```python
from build123d import *

# Parameters (mm, degrees)
SKETCH1_W           = 64.2
SKETCH1_H           = 8.2
SKETCH1_W_2         = 61
SKETCH1_H_2         = 5
BOSS_EXTRUDE1_DEPTH = 90
SKETCH2_W           = 4
SKETCH2_H           = 8.2
BOSS_EXTRUDE2_DEPTH = 2
BOSS_EXTRUDE4_DEPTH = 8
SKETCH5_W           = 17.2
SKETCH5_H           = 27.6
BOSS_EXTRUDE5_DEPTH = 1.6
CHAMFER3_SIZE       = 11
FILLET1_R           = 3
FILLET2_R           = 2
FILLET3_R           = 3
SKETCH3_W           = 10
SKETCH3_H           = 10
BOSS_EXTRUDE3_DEPTH = 0.8


with BuildPart() as part:
    # Sketch1 → Boss-Extrude1 (new body)
    with BuildSketch(Plane.XY):
        Rectangle(SKETCH1_W, SKETCH1_H)
        Rectangle(SKETCH1_W_2, SKETCH1_H_2, mode=Mode.SUBTRACT)
    extrude(amount=BOSS_EXTRUDE1_DEPTH)

    # Sketch2 → Boss-Extrude2 (add)
    with BuildSketch(Plane(origin=(0, 0, 0), x_dir=(-1, 0, 0), z_dir=(0, 0, -1))):
        Rectangle(SKETCH2_W, SKETCH2_H)
    extrude(amount=-BOSS_EXTRUDE2_DEPTH)

    # Sketch4 → Boss-Extrude4 (add)
    with BuildSketch(Plane.XZ.offset(4.1)):
        Polygon((-7, 52.6), (-7, 26.6), (7, 26.6), (7, 52.6), (8.6, 52.6), (8.6, 25), (-8.6, 25), (-8.6, 52.6), align=None)
    extrude(amount=BOSS_EXTRUDE4_DEPTH)

    # Sketch5 → Boss-Extrude5 (add)
    with BuildSketch(Plane.XZ.offset(12.1)):
        with Locations((0, 38.8)):
            Rectangle(SKETCH5_W, SKETCH5_H)
    extrude(amount=BOSS_EXTRUDE5_DEPTH)

    # Chamfer3
    # the kernel refuses this chamfer: 11 mm, written as the material it adds along each edge
    with BuildSketch(Plane(origin=(8.6, -4.1, 25), x_dir=(0, 0.027495876610586372, -0.9996219169112968), z_dir=(-1, 0, 0))) as chamfer3_piece_1_section:
        Polygon((CHAMFER3_SIZE * 0.999621916911, CHAMFER3_SIZE * 0.0274958766106), (-CHAMFER3_SIZE * 0.0274958766106, CHAMFER3_SIZE * 0.999621916911), (0, 0), align=None)
    chamfer3_piece_1 = extrude(amount=17.2, mode=Mode.PRIVATE)
    chamfer3_piece_1 = split(chamfer3_piece_1, bisect_by=Plane(origin=(0, -13.7, 21.279882352), z_dir=(0, 1, 0)), keep=Keep.TOP, mode=Mode.PRIVATE)
    add(chamfer3_piece_1)

    # Fillet1
    fillet1_edges = [part.edges().sort_by_distance(p)[0] for p in [
        (-8.6, -4.1, 33.3),
        (8.6, -4.1, 33.3),
    ]]
    fillet(fillet1_edges, radius=FILLET1_R)

    # Fillet2
    fillet2_edges = [part.edges().sort_by_distance(p)[0] for p in [
        (2, -2.5, 1),
        (-2, -2.5, 1),
        (-2, 2.5, 1),
        (2, 2.5, 1),
    ]]
    fillet(fillet2_edges, radius=FILLET2_R)

    # Fillet3
    fillet3_edges = [part.edges().sort_by_distance(p)[0] for p in [
        (-9.3, -4.1, 52.6),
        (9.3, -4.1, 52.6),
    ]]
    fillet(fillet3_edges, radius=FILLET3_R)

    # Sketch3 → Boss-Extrude3 (add)
    with BuildSketch(Plane(origin=(0, 0, 0), x_dir=(-1, 0, 0), z_dir=(0, 0, -1))):
        with Locations((-35.5, 9.1)):
            Rectangle(SKETCH3_W, SKETCH3_H)
        with Locations((35.5, 9.1)):
            Rectangle(SKETCH3_W, SKETCH3_H)
        with Locations((35.5, -9.1)):
            Rectangle(SKETCH3_W, SKETCH3_H)
        with Locations((-35.5, -9.1)):
            Rectangle(SKETCH3_W, SKETCH3_H)
    extrude(amount=-BOSS_EXTRUDE3_DEPTH)


solid = part.part
```
The listing builds one solid part. Answer for the finished solid, in the listing's coordinates (mm). A direction names the side the tool comes from. Round coordinates to 2 decimals unless told otherwise and drop trailing zeros. Loops run counter-clockwise (first coordinate to the right, second up) from the corner with the lowest first, then second, coordinate; pieces in that order, holes last.
1) Consider line 1 (Y direction, x = -1, z = 28.5); line 2 (Y direction, x = -8, z = 60); line 3 (X direction, y = -10.5, z = 52.5). Determine where each line is inside the solid, lowest interval first.
Outcome:
line 1: y = -13.7 to -12.1, -4.1 to -2.5, 2.5 to 4.1
line 2: y = -4.1 to -2.5, 2.5 to 4.1
line 3: x = -8.6 to -7, 7 to 8.6
2) A cutting plane is placed at B-B on y = 5.75. Determine the outline of the cut face in (x, z).
Outcome:
outline: (-40.5, 0) - (-30.5, 0) - (-30.5, 0.8) - (-40.5, 0.8) - close; (30.5, 0) - (40.5, 0) - (40.5, 0.8) - (30.5, 0.8) - close
3) A cutting plane is placed at A-A on x = 25.5. Determine the outline of the cut face in (y, z).
Outcome:
outline: (-4.1, 0) - (-2.5, 0) - (-2.5, 90) - (-4.1, 90) - close; (2.5, 0) - (4.1, 0) - (4.1, 90) - (2.5, 90) - close
4) A cutting plane is placed at D-D on y = -9.5. Determine the outline of the cut face in (x, z), plus the area to 3 significant figures.
Outcome:
outline: (-40.5, 0) - (-30.5, 0) - (-30.5, 0.8) - (-40.5, 0.8) - close; (-8.6, 19.4) - (8.6, 19.4) - (8.6, 52.6) - (7, 52.6) - (7, 26.6) - (-7, 26.6) - (-7, 52.6) - (-8.6, 52.6) - close; (30.5, 0) - (40.5, 0) - (40.5, 0.8) - (30.5, 0.8) - close
area: 223 mm2
5) For a pull along X with two mould halves and no side action, classify faces 1 (the face through (7, -8, 41)), 2 (the face through (0, -2.5, 44)), 3 (the face through (0, 1, 0)), 4 (the face through (-9.5, -4.96, 34.51)) as released by +X, released by -X, zero draft, split by the parting line, or undercut.
Outcome:
face 1: undercut
face 2: undercut
face 3: zero draft
face 4: released by -X
6) A cutting plane is placed at C-C on z = 30. Determine the outline of the cut face in (x, y), plus the area to 3 significant figures.
Outcome:
outline: (-32.1, -4.1) - (-11.6, -4.1) arc R3 cw to (-8.6, -7.1) - (-8.6, -13.7) - (8.6, -13.7) - (8.6, -7.1) arc R3 cw to (11.6, -4.1) - (32.1, -4.1) - (32.1, 4.1) - (-32.1, 4.1) - close; hole (-30.5, -2.5) - (30.5, -2.5) - (30.5, 2.5) - (-30.5, 2.5) - close; hole (-7, -12.1) - (7, -12.1) - (7, -4.1) - (-7, -4.1) - close
area: 278 mm2
7) For faces 5 (the face through (-8.6, -10, 35)), 6 (the face through (9.5, -4.96, 35.09)), 7 (the face through (-35, -9, 0.8)), 8 (the face through (0, 3, 90)), 9 (the face through (30.5, 0, 44)), determine the directions among +Z, -Z, +X, -X, +Y, -Y from which every point of the face is accessible in a straight line to the end or side of a thin tool.
Outcome:
face 5: +Z, -Z, -X, -Y
face 6: +Z, -Z, +X, -Y
face 7: +Z, +X, -X, -Y
face 8: +Z, +X, -X, +Y, -Y
face 9: +Z, -Z
8) Given P1, Ø6.5, axis at y = -0.5, z = 24, coming from the +X side; P2, Ø2, axis at x = -1.5, y = -10.5, coming from the +Z side; P3, Ø4, axis at y = -7.5, z = 39, coming from the -X side, each flat-ended and moving along its own axis, determine where each tip first touches the part or whether it passes through.
Outcome:
P1: stops at x = 32.1
P2: stops at z = 26.6
P3: stops at x = -9.06
